Verification items for the finished model (mm, model axes). Coordinates: 2 decimals unless noted, no trailing zeros. Order: outer loops, then holes, each group sorted by start corner. A loop starts at its lowest first (then second) coordinate and runs counter-clockwise, first axis right, second up.
Q1. Cross-section at B-B, the plane y = 3.5. Count the separate pieces of the cut face and the enclosed holes in it, and give its area (3 significant figures).
Q2. Thickness scan on line 1 (X direction, y = 0.9, z = 110); line 2 (X direction, y = 2.25, z = 130); line 3 (Y direction, x = 7, z = 8). Record the ranges inside material, lowest first.
Q3. Depth check by flat-ended pin: P1, Ø4.5, axis at x = 4.5, z = 50, coming from the +Y side. Enter the tip coordinate at first touch or a pass-through.
Q4. Cross-section at A-A, the plane z = 50. Record the boundary of the cut face in (x, y).
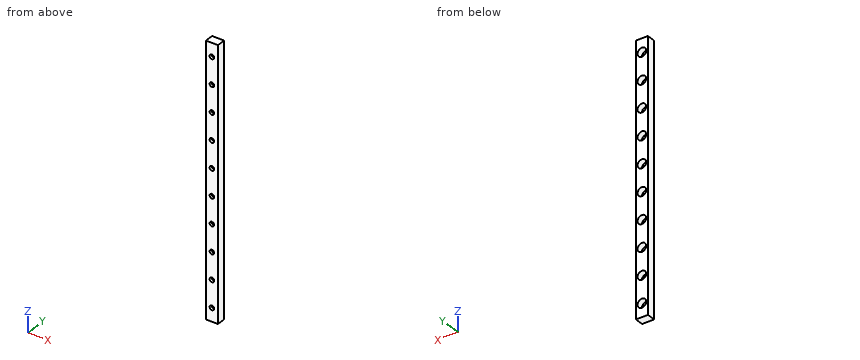
from build123d import *

# Parameters (mm, degrees)
SKETCH1_W                      = 9
SKETCH1_H                      = 6.5
BOSS_EXTRUDE1_DEPTH            = 200
CBORE_FOR_M3_SHCS1_D           = 3.4
CBORE_FOR_M3_SHCS1_CBORE_D     = 6.5
CBORE_FOR_M3_SHCS1_CBORE_DEPTH = 4.5


with BuildPart() as part:
    # Sketch1 → Boss-Extrude1 (new body)
    with BuildSketch(Plane.XY):
        with Locations((4.5, 3.25)):
            Rectangle(SKETCH1_W, SKETCH1_H)
    extrude(amount=BOSS_EXTRUDE1_DEPTH)

    # CBORE for M3 SHCS1 (through all)
    with Locations(Plane(origin=(0, 6.5, 0), x_dir=(1, 0, 0), z_dir=(0, 1, 0))):
        with Locations((4.5, -190), (4.5, -170), (4.5, -150), (4.5, -130), (4.5, -110), (4.5, -90), (4.5, -70), (4.5, -50), (4.5, -30), (4.5, -10)):
            CounterBoreHole(CBORE_FOR_M3_SHCS1_D / 2, CBORE_FOR_M3_SHCS1_CBORE_D / 2, CBORE_FOR_M3_SHCS1_CBORE_DEPTH)


solid = part.part
Check values:
1. separate pieces: 1
1. enclosed holes: 10
1. area: 1,470 mm2
2. line 1: x = 0 to 2.8, 6.2 to 9
2. line 2: x = 0 to 1.25, 7.75 to 9
2. line 3: y = 0 to 2
3. P1: stops at y = 2
4. outline: (0, 0) - (2.8, 0) - (2.8, 2) - (1.25, 2) - (1.25, 6.5) - (0, 6.5) - close; (6.2, 0) - (9, 0) - (9, 6.5) - (7.75, 6.5) - (7.75, 2) - (6.2, 2) - close
